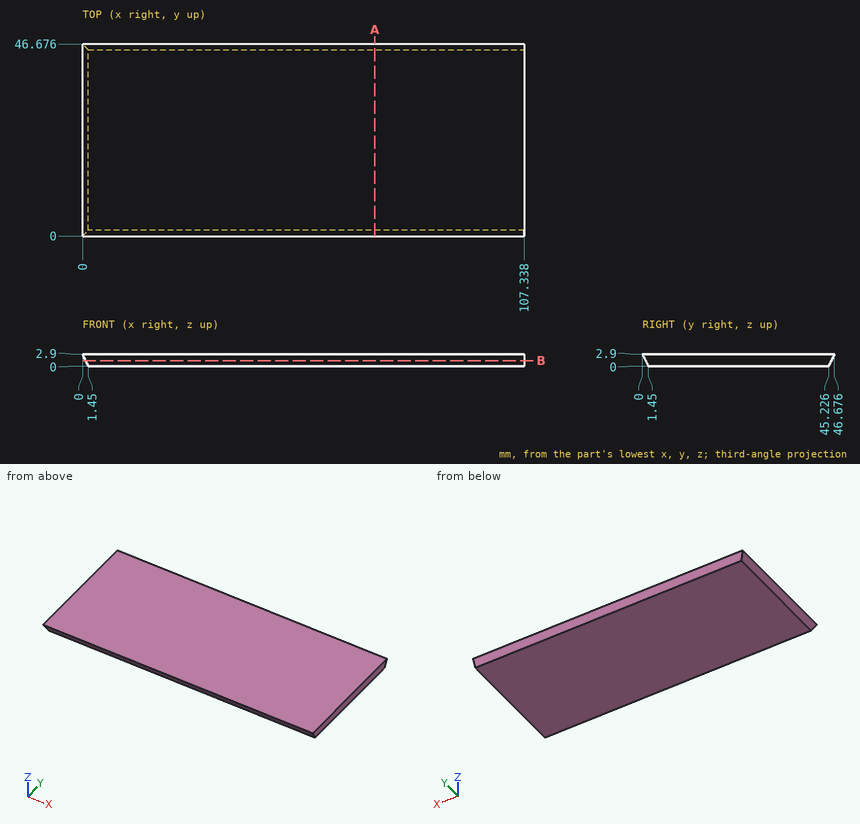
Part print with two shaded views. Sizes in mm from the minimum x, y, z corner. Round coordinates to 2 decimals unless told otherwise and drop trailing zeros. Loops run counter-clockwise (first coordinate to the right, second up) from the corner with the lowest first, then second, coordinate; pieces in that order, holes last. Notation, with made-up numbers: M 41.25,-25 L 47.25,-25 A20 ccw 47.25,-8 Z; hole C 18,-29 d2. An arc over 180 degrees is marked long. Return JSON: item names as keys, results as strings. Group by question number.
(1) Saw through at A-A, the plane x = 71. List the corners of the cut face in (y, z), and give its area (3 significant figures).
(2) Drop flat-ended pins along their axis: P1, Ø10, axis at x = 37, y = 36.5, coming from the -Z side; P2, Ø1.5, axis at x = 20, z = 0.5, coming from the +Y side. Give the stop position or say it passes through.
(3) Saw through at B-B, the plane z = 1.35. List the corners of the cut face in (x, y) (1 decimal).
(4) Wall check: probe 1 along X at (y, z) = (30, 0.2); probe 2 along Y at (x, z) = (45.5, 0.9) (1 decimal); probe 3 along X at (y, z) = (27, 1.75) (1 decimal). Give the ranges that are in metal, low to high. Write a range as [from, to].
Answer list:
{
 "1": {"outline": "M 0,2.9 L 1.45,0 L 45.23,0 L 46.68,2.9 Z", "area": "131 mm2"},
 "2": {"P1": "z = 0", "P2": "y = 45.85"},
 "3": {"outline": "M 0.8,0.8 L 107.3,0.8 L 107.3,45.9 L 0.8,45.9 Z"},
 "4": {"probe 1": "[1.35, 107.34]", "probe 2": "[1, 45.7]", "probe 3": "[0.6, 107.3]"}
}
